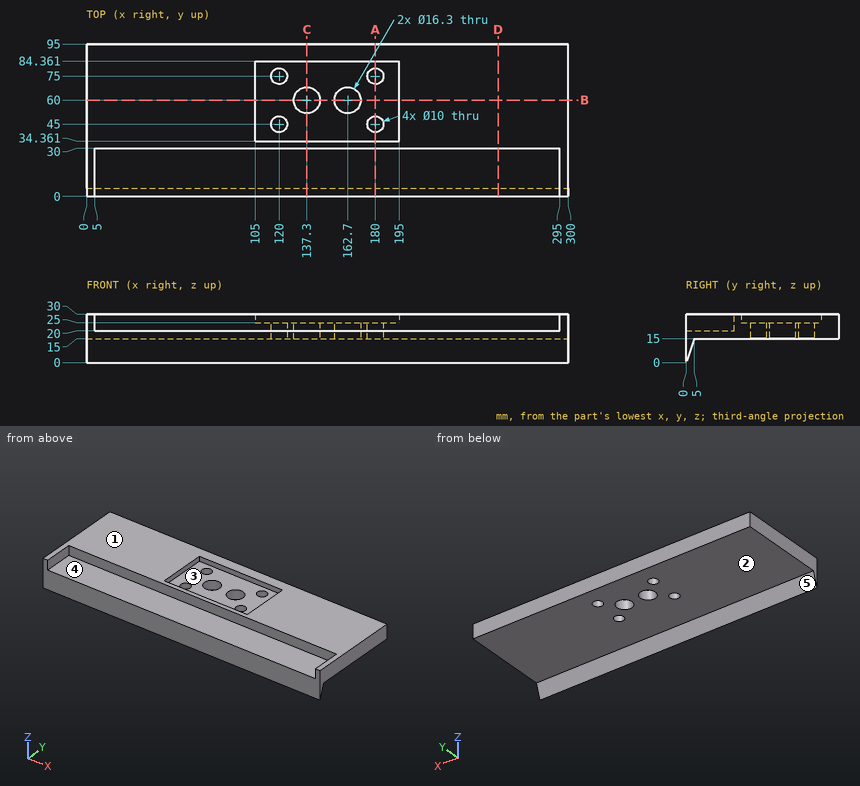
Geometry check sheet. Reference: drawing and pictorial views, mm from the part's lowest x, y, z. A direction names the side the tool comes from. Round coordinates to 2 decimals unless told otherwise and drop trailing zeros. Order: outer loops, then holes, each group sorted by start corner. A loop starts at its lowest first (then second) coordinate and runs counter-clockwise, first axis right, second up. Notation, with made-up numbers: (22, 2.5) - (38, 2.5) arc R19 cw to (38, 12.5) - close; hole circle Ø9 at (-32, 20.5). An arc over 180 degrees is marked (long way). One line per question, with ' | ' between items. Start each with the question number.
(1) Sectioned sample at D-D on x = 256.5. Record the cut outline in (y, z), and give its area (3 significant figures).
(2) Depth check by flat-ended pin: pin 1 Ø12 at (x, z) = (179.5, 8) entering from +Y; pin 2 Ø13 at (x, y) = (137.3, 60) entering from -Z; pin 3 Ø24 at (x, y) = (166.5, 15.5) entering from +Z; pin 4 Ø21 at (x, y) = (162.7, 60) entering from +Z. Enter the tip coordinate at first touch or a pass-through.
(3) Sectioned sample at A-A on x = 180. Record the cut outline in (y, z).
(4) Sectioned sample at B-B on y = 60. Record the cut outline in (x, z), and give its area (3 significant figures).
(5) Release check for a two-part mould opening along X. For the marked faces 4 and 5 record: released by +X, released by -X, zero draft, split by the parting line, or undercut.
(6) Access from +Z, -Z, +X, -X, +Y, -Y to the whole of each face (thin tool, end or side, straight path). Record for the marked faces 1, 2 and 3.
(7) Thickness scan on L1, parallel to Y at x = 180, z = 22; L2, parallel to Y at x = 120, z = 19.25; L3, parallel to Y at x = 162.7, z = 22.5. Record the ranges inside material, lowest first. Write a range as [from, to].
(8) Sectioned sample at C-C on x = 137.3. Record the cut outline in (y, z).
Conclusion:
1) outline: (0, 0) - (5, 15) - (95, 15) - (95, 30) - (30, 30) - (30, 20) - (0, 20) - close | area: 1,160 mm2
2) pin 1: stops at y = 4.67 | pin 2: passes through | pin 3: stops at z = 20 | pin 4: stops at z = 25
3) outline: (0, 0) - (5, 15) - (40, 15) - (40, 25) - (34.36, 25) - (34.36, 30) - (30, 30) - (30, 20) - (0, 20) - close; (50, 15) - (70, 15) - (70, 25) - (50, 25) - close; (80, 15) - (95, 15) - (95, 30) - (84.36, 30) - (84.36, 25) - (80, 25) - close
4) outline: (0, 15) - (129.15, 15) - (129.15, 25) - (105, 25) - (105, 30) - (0, 30) - close; (145.45, 15) - (154.55, 15) - (154.55, 25) - (145.45, 25) - close; (170.85, 15) - (300, 15) - (300, 30) - (195, 30) - (195, 25) - (170.85, 25) - close | area: 3,720 mm2
5) face 4: undercut | face 5: zero draft
6) face 1: +Z, +X, -X, +Y, -Y | face 2: -Z, +X, -X, +Y | face 3: +Z
7) L1: y = [30, 40], [50, 70], [80, 95] | L2: y = [0, 40], [50, 70], [80, 95] | L3: y = [30, 51.85], [68.15, 95]
8) outline: (0, 0) - (5, 15) - (51.85, 15) - (51.85, 25) - (34.36, 25) - (34.36, 30) - (30, 30) - (30, 20) - (0, 20) - close; (68.15, 15) - (95, 15) - (95, 30) - (84.36, 30) - (84.36, 25) - (68.15, 25) - close
